from build123d import *

# Parameters (mm, degrees)
BOSS_EXTRUDE1_DEPTH = 4.7625
SKETCH2_R           = 2.54
SKETCH2_R_2         = 1.143
CUT_EXTRUDE1_DEPTH  = 89.827590344


with BuildPart() as part:
    # Sketch1 → Boss-Extrude1 (new body)
    with BuildSketch(Plane.XY):
        with BuildLine():
            Line((-77.310617813, 19.05), (-47.689382187, 19.05))
            ThreePointArc((-47.689382187, 19.05), (0, 12.7), (47.689382187, 19.05))
            Line((47.689382187, 19.05), (77.310617813, 19.05))
            ThreePointArc((77.310617813, 19.05), (86.63, 0), (77.310617813, -19.05))
            Line((77.310617813, -19.05), (47.689382187, -19.05))
            ThreePointArc((47.689382187, -19.05), (0, -12.7), (-47.689382187, -19.05))
            Line((-47.689382187, -19.05), (-77.310617813, -19.05))
            ThreePointArc((-77.310617813, -19.05), (-86.63, 0), (-77.310617813, 19.05))
        make_face()
    extrude(amount=BOSS_EXTRUDE1_DEPTH)

    # Sketch2 → Cut-Extrude1 (cut, through all)
    with BuildSketch(Plane.XY.offset(4.7625)):
        with Locations((-62.5, 0)):
            Circle(SKETCH2_R)
        with Locations((-54.118, 0)):
            Circle(SKETCH2_R_2)
        with Locations((-62.5, -8.382)):
            Circle(SKETCH2_R_2)
        with Locations((-70.882, 0)):
            Circle(SKETCH2_R_2)
        with Locations((-62.5, 8.382)):
            Circle(SKETCH2_R_2)
        with Locations((62.5, 0)):
            Circle(SKETCH2_R)
        with Locations((70.882, 0)):
            Circle(SKETCH2_R_2)
        with Locations((62.5, -8.382)):
            Circle(SKETCH2_R_2)
        with Locations((54.118, 0)):
            Circle(SKETCH2_R_2)
        with Locations((62.5, 8.382)):
            Circle(SKETCH2_R_2)
    extrude(amount=-CUT_EXTRUDE1_DEPTH, mode=Mode.SUBTRACT)


solid = part.part
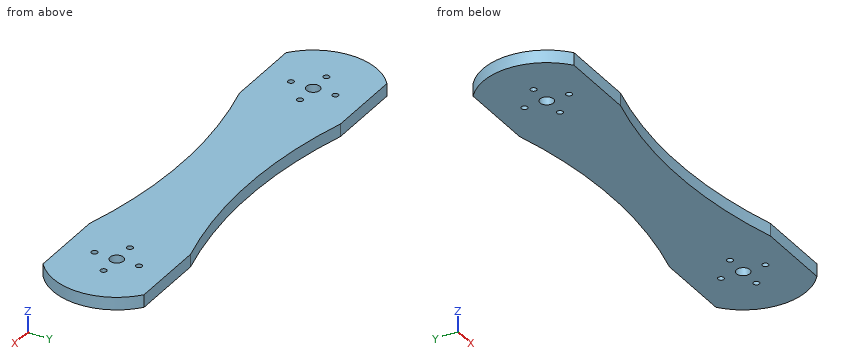
Verification items for the finished model (mm, model axes). Coordinates: 2 decimals unless noted, no trailing zeros. Loops run counter-clockwise (first coordinate to the right, second up) from the corner with the lowest first, then second, coordinate; pieces in that order, holes last. Notation, with made-up numbers: (-35, -5) -> (-15, -5) arc R24 cw to (-15, 28) -> close; hole circle Ø3 at (35.25, -22.5). An arc over 180 degrees is marked (long way). Answer as a JSON object with one key per item and string values. Group by question number.
Item 1: Depth check by flat-ended pin: pin 1 (2 mm diameter, centred on y = 0.5, z = 1, fed in from -X). Enter the tip coordinate at first touch or a pass-through.
Item 2: Scan lines: probe 1 along Y at (x, z) = (62.5, 1.05) (3 decimals); probe 2 along X at (y, z) = (-8.5, 4.4); probe 3 along Y at (x, z) = (62, 2.1). Record each from-to range of solid material in increasing order.
Item 3: Sectioned sample at A-A on y = -14.5. Record the boundary of the cut face in (x, z), plus the area to 3 significant figures.
Item 4: Sectioned sample at D-D on y = 17.5. Record the boundary of the cut face in (x, z).
Item 5: Sectioned sample at C-C on x = -5. Record the boundary of the cut face in (y, z).
Item 6: Sectioned sample at B-B on z = 3.65. State how many separate pieces and enclosed holes the cut face has, plus the area to 3 significant figures.
Evaluation:
{
 "1": {"pin 1": "stops at x = -86.63"},
 "2": {"probe 1": "y = -19.05 to -9.525, -7.239 to -2.54, 2.54 to 7.239, 9.525 to 19.05", "probe 2": "x = -85.08 to -63.64, -61.36 to 61.36, 63.64 to 85.08", "probe 3": "y = -19.05 to -9.41, -7.35 to -2.49, 2.49 to 7.35, 9.41 to 19.05"},
 "3": {"outline": "(-81.79, 0) -> (-25.55, 0) -> (-25.55, 4.76) -> (-81.79, 4.76) -> close; (25.55, 0) -> (81.79, 0) -> (81.79, 4.76) -> (25.55, 4.76) -> close", "area": "536 mm²"},
 "4": {"outline": "(-79.11, 0) -> (-41.55, 0) -> (-41.55, 4.76) -> (-79.11, 4.76) -> close; (41.55, 0) -> (79.11, 0) -> (79.11, 4.76) -> (41.55, 4.76) -> close"},
 "5": {"outline": "(-12.77, 0) -> (12.77, 0) -> (12.77, 4.76) -> (-12.77, 4.76) -> close"},
 "6": {"separate pieces": "1", "enclosed holes": "10", "area": "5,500 mm²"}
}
